Build history of the part. All positions in model axes, mm. A direction names the side the tool comes from. Round coordinates to 2 decimals unless told otherwise and drop trailing zeros. Loops run counter-clockwise (first coordinate to the right, second up) from the corner with the lowest first, then second, coordinate; pieces in that order, holes last. Notation, with made-up numbers: M 55,32.5 L 92,32.5 A35 ccw 92,67.5 Z; hole C 68,-38 d10. An arc over 180 degrees is marked long. Write each question's results on one line, items separated by ' | '. Start each with the question number.
```python
from build123d import *

# Parameters (mm, degrees)
SKETCH1_W               = 50.8
SKETCH1_H               = 96.5708
BOSS_EXTRUDE1_DEPTH     = 101.6
CUT_EXTRUDE1_DEPTH      = 143.455745453
CUT_EXTRUDE1_DEPTH_BACK = 25.4
FILLET1_R               = 12.7
FILLET2_R               = 12.7
SKETCH4_W               = 50.8
SKETCH4_H               = 4
BOSS_EXTRUDE2_DEPTH     = 25.4
BOSS_EXTRUDE3_DEPTH     = 4
M4_CLEARANCE_HOLE1_D    = 4.5
MIRROR2_COPY_1_DEPTH    = 4
SKETCH10_W              = 19.05
SKETCH10_H              = 57.15
CUT_EXTRUDE2_DEPTH      = 95.25
FILLET3_R               = 2


with BuildPart() as part:
    # Sketch1 → Boss-Extrude1 (new body)
    with BuildSketch(Plane.XY):
        Rectangle(SKETCH1_W, SKETCH1_H)
    extrude(amount=BOSS_EXTRUDE1_DEPTH)

    # Sketch2 → Cut-Extrude1 (cut, two sides: drawn at the far end of the back side and taken through both)
    with BuildSketch(Plane.XZ.offset(48.2854).offset(-CUT_EXTRUDE1_DEPTH_BACK)):
        with BuildLine():
            Line((-25.4, 0), (-3.175, 0))
            ThreePointArc((-3.175, 0), (-6.041573742, 48.089456834), (-15.875, 95.25))
            Line((-15.875, 95.25), (-25.4, 95.25))
            Line((-25.4, 95.25), (-25.4, 0))
        make_face()
        with BuildLine():
            ThreePointArc((15.875, 95.25), (6.041573742, 48.089456834), (3.175, 0))
            Line((3.175, 0), (25.4, 0))
            Line((25.4, 0), (25.4, 95.25))
            Line((25.4, 95.25), (15.875, 95.25))
        make_face()
    extrude(amount=CUT_EXTRUDE1_DEPTH + CUT_EXTRUDE1_DEPTH_BACK, mode=Mode.SUBTRACT)

    # Fillet1
    fillet1_edges = [part.edges().sort_by_distance(p)[0] for p in [
        (6.041573742, -22.8854, 48.089456834),
        (-6.041573742, -22.8854, 48.089456834),
    ]]
    fillet(fillet1_edges, radius=FILLET1_R)

    # Fillet2
    # the kernel refuses this fillet: 12.7 mm, written as the material it adds along each edge
    with BuildSketch(Plane(origin=(-15.875, -48.2854, 95.25), x_dir=(-1, 0, 0), z_dir=(0, 1, 0))) as fillet2_piece_1:
        with BuildLine():
            CenterArc((9.726246489, -12.698405406), FILLET2_R, 90.90795725, 74.851551617)
            Line((-2.583504713, -9.57430148), (-2.829699737, -9.511819402))
            ThreePointArc((-2.829699737, -9.511819402), (-1.57292596, -4.711279583), (-0.244207713, 0.069846926))
            Line((-0.244207713, 0.069846926), (0, 0.254))
            ThreePointArc((0, 0.254), (4.7625, 0.254), (9.52097507, 0.253968108))
            Line((9.52097507, 0.253968108), (9.525, 0))
        make_face()
    extrude(amount=37.491851666)
    with BuildSketch(Plane(origin=(15.875, -48.2854, 95.25), x_dir=(1, 0, 0), z_dir=(0, 1, 0))) as fillet2_piece_2:
        with BuildLine():
            CenterArc((9.726246489, 12.698405406), FILLET2_R, 194.240491133, 74.851551617)
            Line((-2.583504713, 9.57430148), (-2.829699737, 9.511819402))
            ThreePointArc((-2.829699737, 9.511819402), (-1.57292596, 4.711279583), (-0.244207713, -0.069846926))
            Line((-0.244207713, -0.069846926), (0, -0.254))
            ThreePointArc((0, -0.254), (4.7625, -0.254), (9.52097507, -0.253968108))
            Line((9.52097507, -0.253968108), (9.525, 0))
        make_face()
    extrude(amount=37.491851666)

    # Sketch4 → Boss-Extrude2 (add)
    with BuildSketch(Plane.XY.offset(101.6)):
        with Locations((0, -46.2854)):
            Rectangle(SKETCH4_W, SKETCH4_H)
    boss_extrude2 = extrude(amount=BOSS_EXTRUDE2_DEPTH)

    # Sketch5 → Boss-Extrude3 (add)
    with BuildSketch(Plane(origin=(25.4, 0, 0), x_dir=(0, 0, -1), z_dir=(1, 0, 0))):
        Polygon((-101.6, -28.4104), (-127, -44.2854), (-101.6, -44.2854), align=None)
    boss_extrude3 = extrude(amount=-BOSS_EXTRUDE3_DEPTH)

    # Mirror1: Boss-Extrude3 across plane
    add(boss_extrude3.mirror(Plane(origin=(0, 0, 0), x_dir=(0, 0, 1), z_dir=(1, 0, 0))))

    # M4 Clearance Hole1 (through all)
    with Locations(Plane(origin=(0, -44.2854, 0), x_dir=(1, 0, 0), z_dir=(0, 1, 0))):
        with Locations((-10.7, -114.3), (10.7, -114.3)):
            m4_clearance_hole1 = Hole(M4_CLEARANCE_HOLE1_D / 2)

    # Mirror2: Boss-Extrude2, Boss-Extrude3, M4 Clearance Hole1 across plane
    add(boss_extrude2.mirror(Plane.ZX))
    add(boss_extrude3.mirror(Plane.ZX))
    add(m4_clearance_hole1.mirror(Plane.ZX), mode=Mode.SUBTRACT)

    # Mirror2 copy 1 sketch → Mirror2 copy 1 (add)
    with BuildSketch(Plane(origin=(-25.4, 0, 0), x_dir=(0, 0, -1), z_dir=(-1, 0, 0))):
        Polygon((-101.6, -28.4104), (-127, -44.2854), (-101.6, -44.2854), align=None)
    extrude(amount=-MIRROR2_COPY_1_DEPTH)

    # Sketch10 → Cut-Extrude2 (cut)
    with BuildSketch(Plane(origin=(0, 0, 0), x_dir=(-1, 0, 0), z_dir=(0, 0, -1))):
        with Locations((-15.875, 19.7104)):
            Rectangle(SKETCH10_W, SKETCH10_H)
        with Locations((15.875, 19.7104)):
            Rectangle(SKETCH10_W, SKETCH10_H)
    extrude(amount=-CUT_EXTRUDE2_DEPTH, mode=Mode.SUBTRACT)

    # Fillet3
    fillet3_edges = [part.edges().sort_by_distance(p)[0] for p in [
        (6.35, -8.8646, 47.625),
        (6.35, 19.7104, 95.25),
        (15.875, -8.8646, 95.25),
        (-6.35, -8.8646, 47.625),
        (-15.875, -8.8646, 95.25),
        (-6.35, 19.7104, 95.25),
    ]]
    fillet(fillet3_edges, radius=FILLET3_R)


solid = part.part
```
Item 1: Saw through at B-B, the plane z = 114.3. State how many separate pieces and enclosed holes the cut face has, then the cut area to 3 significant figures.
Item 2: Drop flat-ended pins along their axis: pin 1 (8.5 mm diameter, centred on x = 19.5, y = 27, fed in from -Z); pin 2 (7.5 mm diameter, centred on x = -20, z = 45.5, fed in from -Y); pin 3 (7.5 mm diameter, centred on x = 19.5, z = 23, fed in from -Y); pin 4 (17.5 mm diameter, centred on y = -32.5, z = 118.5, fed in from -X). Give the stop position or say it passes through.
Item 3: Drill centre lines: line 1 along X through (y, z) = (-47, 114); line 2 along Z through (x, y) = (10.7, 47.1); line 3 along Z through (x, y) = (-6, 16.5). Where is each one in solid material? Low to high. Write a range as [from, to].
Item 4: Saw through at D-D, the plane y = 31. Give the cut face in (x, z).
Item 5: Tool access for faces 1 (the flat face through (-17, -8.865, 46)), 2 (the cylindrical face through (-17.82, -38.78, 92.59)), 3 (the flat face through (21.4, -40, 109)), 4 (the flat face through (-23.428, -36.237, 114.122)), 5 (the flat face through (17, -8.865, 46)): list every direction of +Z, -Z, +X, -X, +Y, -Y with a clear straight run to the whole face (end or side of a thin tool).
Item 6: Saw through at A-A, the plane y = 4. Give the cut face in (x, z), then the cut area to 3 significant figures.
Item 7: Mould opens along X. For faces 6 (the cylindrical face through (-5.353, -41.847, 42.568)), 7 (the flat face through (22, -22.885, 32)), 8 (the flat face through (0, 44.285, 114)) say: released by +X, released by -X, zero draft, split by the parting line, or undercut.
Working result:
1) separate pieces: 6 | enclosed holes: 0 | area: 461 mm²
2) pin 1: stops at z = 95.25 | pin 2: stops at y = -23.09 | pin 3: stops at y = -22.9 | pin 4: stops at x = -25.4
3) line 1: x = [-25.4, -12.93], [-8.47, 8.47], [12.93, 25.4] | line 2: z = [95.25, 112.05], [116.55, 127] | line 3: z = [0, 101.6]
4) outline: M -25.4,95.25 L -8.35,95.25 A2 cw -6.35,93.25 L -6.35,0 L 6.35,0 L 6.35,93.25 A2 cw 8.35,95.25 L 25.4,95.25 L 25.4,105.74 L 21.4,105.74 L 21.4,101.6 L -21.4,101.6 L -21.4,105.74 L -25.4,105.74 Z
5) face 1: -Z, -X, +Y | face 2: -Z, -X, -Y | face 3: +Z | face 4: +Z, +X, -X | face 5: -Z, +X, +Y
6) outline: M -25.4,95.25 L -8.35,95.25 A2 cw -6.35,93.25 L -6.35,0 L 6.35,0 L 6.35,93.25 A2 cw 8.35,95.25 L 25.4,95.25 L 25.4,101.6 L -25.4,101.6 Z | area: 1,530 mm²
7) face 6: released by -X | face 7: zero draft | face 8: undercut
